```python
from build123d import *

# Parameters (mm, degrees)
EXTRUDE_1_DEPTH          = 5
SKETCH_3_R               = 2.025
CUT_EXTRUDE_1_DEPTH      = 1
CUT_EXTRUDE_1_DEPTH_BACK = 6
FILLET_1_R               = 3
SKETCH_4_R               = 1.525
CUT_EXTRUDE_2_DEPTH      = 1
CUT_EXTRUDE_2_DEPTH_BACK = 6
CUT_EXTRUDE_3_DEPTH      = 6
FILLET_2_R               = 2
SKETCH_8_R               = 7.5
CUT_EXTRUDE_4_DEPTH      = 5


with BuildPart() as part:
    # 草图1 → 凸台-拉伸1 (new body)
    with BuildSketch(Plane.XY):
        Polygon((0, 0), (-55, 0), (-55, -30), (30, -30), (30, 50), (0, 50), align=None)
    extrude(amount=EXTRUDE_1_DEPTH)

    # 草图3 → 切除-拉伸1 (cut, two sides)
    with BuildSketch(Plane(origin=(0, 0, 0), x_dir=(-1, 0, 0), z_dir=(0, 0, -1))) as cut_extrude_1_sk:
        with Locations((-24, 38)):
            Circle(SKETCH_3_R)
        with Locations((-6, 38)):
            Circle(SKETCH_3_R)
        with Locations((-24, 8)):
            Circle(SKETCH_3_R)
        with Locations((-6, 8)):
            Circle(SKETCH_3_R)
    extrude(amount=CUT_EXTRUDE_1_DEPTH, mode=Mode.SUBTRACT)
    extrude(cut_extrude_1_sk.sketch, amount=-CUT_EXTRUDE_1_DEPTH_BACK, mode=Mode.SUBTRACT)

    # 圆角1
    fillet_1_edges = [part.edges().sort_by_distance(p)[0] for p in [
        (0, 50, 2.5),
        (30, 50, 2.5),
        (30, -30, 2.5),
        (-55, -30, 2.5),
        (-55, 0, 2.5),
        (0, 0, 2.5),
    ]]
    fillet(fillet_1_edges, radius=FILLET_1_R)

    # 草图4 → 切除-拉伸2 (cut, two sides)
    with BuildSketch(Plane.XY.offset(5)) as cut_extrude_2_sk:
        with Locations((-48, -25.8)):
            Circle(SKETCH_4_R)
        with Locations((-48, -4.2)):
            Circle(SKETCH_4_R)
        with Locations((-28, -4.2)):
            Circle(SKETCH_4_R)
        with Locations((-28, -25.8)):
            Circle(SKETCH_4_R)
    extrude(amount=CUT_EXTRUDE_2_DEPTH, mode=Mode.SUBTRACT)
    extrude(cut_extrude_2_sk.sketch, amount=-CUT_EXTRUDE_2_DEPTH_BACK, mode=Mode.SUBTRACT)

    # 草图7 → 切除-拉伸3 (cut, through all)
    with BuildSketch(Plane.XY.offset(5)):
        Polygon((13.157303163, -5), (-21, -5), (-21, -21.662099104), align=None)
        Polygon((20, -25), (20, -8.337900896), (-14.157303163, -25), align=None)
    extrude(amount=-CUT_EXTRUDE_3_DEPTH, mode=Mode.SUBTRACT)

    # 圆角2
    fillet_2_edges = [part.edges().sort_by_distance(p)[0] for p in [
        (-14.157303163, -25, 2.5),
        (20, -8.337900896, 2.5),
        (20, -25, 2.5),
        (-21, -21.662099104, 2.5),
        (-21, -5, 2.5),
        (13.157303163, -5, 2.5),
    ]]
    fillet(fillet_2_edges, radius=FILLET_2_R)

    # 草图8 → 切除-拉伸4 (cut)
    with BuildSketch(Plane.XY.offset(5)):
        with Locations((15, 23)):
            Circle(SKETCH_8_R)
    extrude(amount=-CUT_EXTRUDE_4_DEPTH, mode=Mode.SUBTRACT)


solid = part.part
```
Geometry check sheet. Reference: the model listing, model coordinates, mm. A direction names the side the tool comes from. Round coordinates to 2 decimals unless told otherwise and drop trailing zeros. Loops run counter-clockwise (first coordinate to the right, second up) from the corner with the lowest first, then second, coordinate; pieces in that order, holes last. Notation, with made-up numbers: (29, 1.5) - (88, 1.5) arc R12 cw to (88, 17.5) - close; hole circle Ø10 at (28, 24). An arc over 180 degrees is marked (long way). Write each question's results on one line, items separated by ' | '. Start each with the question number.
Q1. Cross-section at D-D on y = 8. Enter the section's corners in (x, z) (3 decimals).
Q2. Access from +Z, -Z, +X, -X, +Y, -Y to the whole of each face (thin tool, end or side, straight path). Record for faces 1 (the flat face through (6, -25, 3)), 2 (the flat face through (0, 25, 2)), 3 (the cylindrical face through (29.1, 49.14, 2.54)).
Q3. Release check for a two-part mould opening along Y. For faces 4 (the flat face through (15, 50, 2)), 5 (the flat face through (30, 9, 2)), 6 (the cylindrical face through (-20.4, -5.57, 2.46)) record: +Y half, -Y half, draft (parallel to the pull), parting line (faces both ways), or undercut.
Q4. Thickness scan on line 1 (Y direction, x = -28, z = 2.6) (3 decimals); line 2 (Y direction, x = 24, z = 3.5) (3 decimals); line 3 (Y direction, x = 6, z = 3.7) (3 decimals). Record the ranges inside material, lowest first. Write a range as [from, to].
Q5. Cross-section at B-B on y = 23. Enter the section's corners in (x, z), and give its area (3 significant figures).
Q6. Gauge pin test, flat ends, axial feed: P1, Ø5, axis at x = -28, y = -4.2, coming from the +Z side; P2, Ø3, axis at x = 6, y = 8, coming from the +Z side (3 decimals); P3, Ø3, axis at y = 38.5, z = 1, coming from the -X side. Record the tip position at first contact, or that the pin passes through.
Q7. Cross-section at C-C on z = 3.6. State how many separate pieces and enclosed holes the cut face has, and give its area (3 significant figures).
Q8. Cross-section at A-A on x = -48. Enter the section's corners in (y, z) (3 decimals).
Answers below:
1) outline: (0, 0) - (3.975, 0) - (3.975, 5) - (0, 5) - close; (8.025, 0) - (21.975, 0) - (21.975, 5) - (8.025, 5) - close; (26.025, 0) - (30, 0) - (30, 5) - (26.025, 5) - close
2) face 1: +Z, -Z | face 2: +Z, -Z, -X, +Y | face 3: +Z, -Z, +X, +Y
3) face 4: +Y half | face 5: draft | face 6: undercut
4) line 1: y = [-30, -27.325], [-24.275, -5.725], [-2.675, 0] | line 2: y = [-30, 5.975], [10.025, 35.975], [40.025, 50] | line 3: y = [-30, -25], [-15.167, -8.318], [-5.682, 5.975], [10.025, 35.975], [40.025, 50]
5) outline: (0, 0) - (7.5, 0) - (7.5, 5) - (0, 5) - close; (22.5, 0) - (30, 0) - (30, 5) - (22.5, 5) - close | area: 75.0 mm²
6) P1: stops at z = 5 | P2: passes through | P3: stops at x = 0
7) separate pieces: 1 | enclosed holes: 11 | area: 3,250 mm²
8) outline: (-30, 0) - (-27.325, 0) - (-27.325, 5) - (-30, 5) - close; (-24.275, 0) - (-5.725, 0) - (-5.725, 5) - (-24.275, 5) - close; (-2.675, 0) - (0, 0) - (0, 5) - (-2.675, 5) - close
